Geometry: see drawing. Coordinates: mm, zero at the bounding-box minimum. A direction names the side the tool comes from. Give positions to 0.01 mm unless a question says otherwise; leave off trailing zeros. Order: outer loops, then holes, each group sorted by start corner. A loop starts at its lowest first (then second) coordinate and runs counter-clockwise, first axis right, second up. Notation, with made-up numbers: (-31, 6) - (16, 6) arc R26 ccw to (16, 20) - close; hole circle Ø4 at (50, -13). An arc over 180 degrees is marked (long way). One line per question, with ' | ' between items. Start each with the question number.
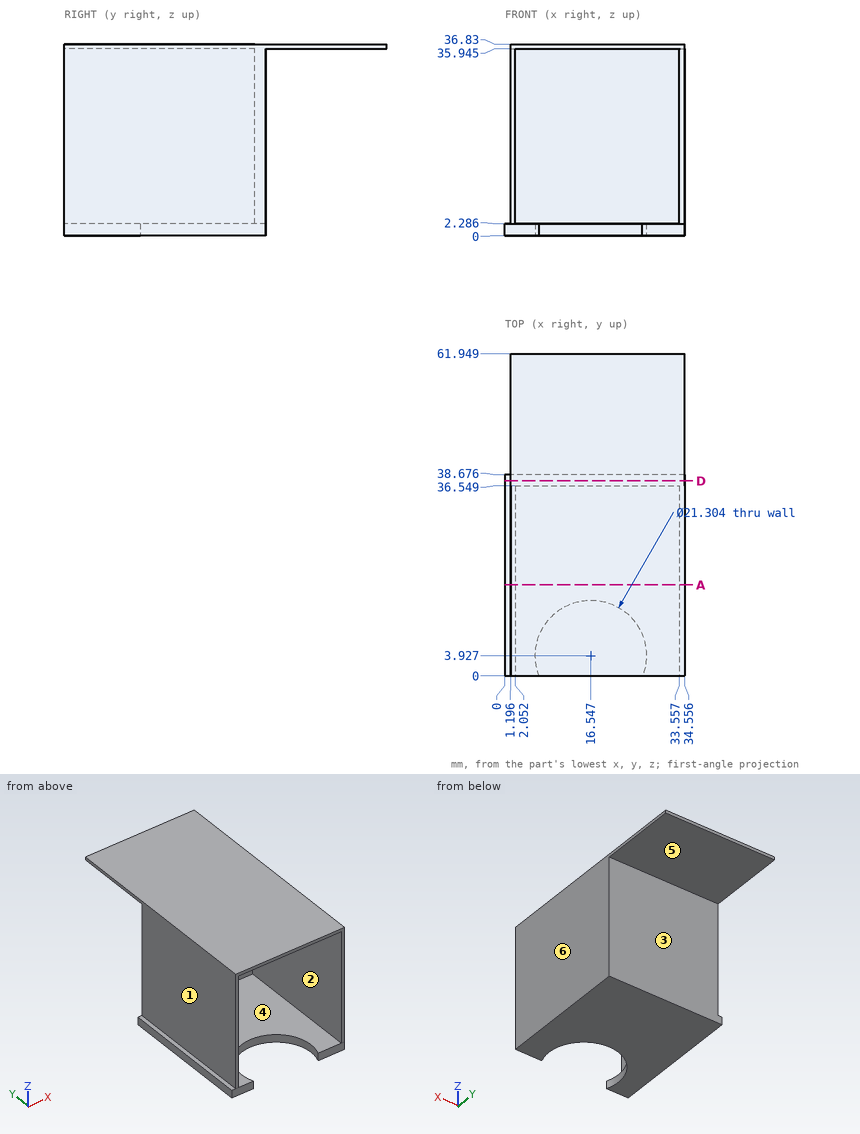
(1) Cut plane A-A, the plane y = 17.5. Return the cut outline in (x, z) (1 decimal), plus the area to 3 significant figures.
(2) Material intervals for line 1 along X through (y, z) = (35, 11) (1 decimal); line 2 along Z through (x, y) = (33, 5.5) (1 decimal); line 3 along Y through (x, z) = (11, 7), sorted ascending. Write a range as from..to.
(3) Pull-direction query (Z, two-part tool) for the marked faces 4, 5 and 6; classes: +Z half, -Z half, draft (parallel to the pull), parting line (faces both ways), or undercut.
(4) Access query for the marked faces 1, 2 and 3. Directions: +Z, -Z, +X, -X, +Y, -Y. A direction counts if a zero-diameter tool reaches every point of the face in a straight line with its end or side. Return the directions, or none.
(5) Cut plane D-D, the plane y = 37.5. Return the cut outline in (x, z) (1 decimal).
(6) Contact query for flat-ended pins moving along their axis: P1, Ø10.5, axis at x = 17.5, z = 17.5, coming from the +Y side; P2, Ø10, axis at y = 33, z = 25.5, coming from the -X side; P3, Ø2, axis at x = 7, z = 25.5, coming from the -Y side. Output: stop coordinate, or through.
Results are:
1) outline: (0, 0) - (34.6, 0) - (34.6, 36.8) - (1.2, 36.8) - (1.2, 2.3) - (0, 2.3) - close; hole (2.1, 2.3) - (33.6, 2.3) - (33.6, 35.9) - (2.1, 35.9) - close | area: 171 mm2
2) line 1: 1.2..2.1, 33.6..34.6 | line 2: 0..2.3, 35.9..36.8 | line 3: 36.55..38.68
3) face 4: undercut | face 5: -Z half | face 6: draft
4) face 1: +Z, -X, +Y, -Y | face 2: -Y | face 3: -Z, +X, -X, +Y
5) outline: (0, 0) - (34.6, 0) - (34.6, 36.8) - (1.2, 36.8) - (1.2, 2.3) - (0, 2.3) - close
6) P1: y = 38.68 | P2: x = 1.2 | P3: y = 36.55
